Geometry: final body of the model. Coordinates: model frame, mm. Face numbers are marked on the shaded views. A direction names the side the tool comes from. Give positions to 0.01 mm unless a question says otherwise; leave off trailing zeros. Write each loop counter-clockwise with the first axis right and the second up, starting at its lowest first coordinate (ties: lowest second). Pieces come first, ordered by that corner, then holes.
Q1. Cut plane B-B on x = -4. Return the cut outline in (y, z), plus the area to 3 significant figures.
Q2. Cut plane D-D on y = -9.25. Return the cut outline in (x, z), plus the area to 3 significant figures.
Q3. Pin query (flat end, axial travel): pin 1 (10 mm diameter, centred on x = -4, z = -16, fed in from +Y); pin 2 (1 mm diameter, centred on x = -10, z = -24, fed in from -Y); pin 3 (3 mm diameter, centred on y = 8, z = -17, fed in from -X); pin 4 (8 mm diameter, centred on x = -11, y = 3, fed in from +Z). Return the tip coordinate at first contact, or that it passes through.
Q4. Cut plane C-C on y = -2. Return the cut outline in (x, z), plus the area to 3 significant figures.
Q5. Reachability of the marked faces 4, 5 and 6 from +Z, -Z, +X, -X, +Y, -Y: full face, straight path, thin tool, end or side. Return the list, or none.
Q6. Line query: L1, parallel to Y at x = 0, z = -24.5; L2, parallel to Z at x = -4, y = 16.5; L3, parallel to Y at x = -17, z = -4. Output: solid intervals per line, ascending.
Q7. Draft query along Y for the marked faces 1, 2 and 3. Return one class per face: pulls with the +Y half, pulls with the -Y half, needs draft (parallel to the pull), parting line crosses it, or undercut.
Q8. Cut plane A-A on z = -16. Return the cut outline in (x, y).
Autodesk Inventor part; units mm, degrees
ref_plane "Work Plane1" through (-15, 0, -27.5) normal (-1, 0, 0) x (0, -1, 0)
ref_plane "YZ Plane" through (0, 0, 0) normal (1, 0, 0) x (0, 1, 0)
ref_plane "XZ Plane" through (0, 0, 0) normal (0, 1, 0) x (-1, 0, 0)
sketch "Sketch1" plane through (0, 0, 0) normal (0, 1, 0) x (-1, 0, 0)
  line L0 (0, 0) -> (-25, 0)
  line L1 (-25, 0) -> (-25, -10)
  line L2 (-25, -10) -> (-15, -10)
  line L3 (-15, -10) -> (-15, -45)
  line L4 (-15, -45) -> (0, -45)
  line L5 (0, 0) -> (0, -45)
  dimension "d3" = 25
  dimension "d4" = 10
  dimension "d5" = 10
  dimension "d6" = 35
  dimension "d7" = 15
revolve "Revolution1" add sketch "Sketch1" angle 360 about axis through (0, 0, 0) along (0, 0, -1)
sketch "Sketch2" plane through (0, 0, 0) normal (0, 0, 1) x (1, 0, 0)
  line L0 (0, 0) -> (30.242, 0) construction
  line L1 (0, 0.5707) -> (22.435, 0.5707) construction
  circle A0 centre (9.7519, 17.4614) radius 2.25
  circle A1 centre (19.998, 0.2854) radius 2.25
  circle A2 centre (10.2461, -17.1761) radius 2.25
  circle A3 centre (-9.7519, -17.4614) radius 2.25
  circle A4 centre (-19.998, -0.2854) radius 2.25
  circle A5 centre (-10.2461, 17.1761) radius 2.25
  dimension "d12" = 4.5
  dimension "d15" = 360
extrude "Extrusion1" cut sketch "Sketch2" against normal through all
sketch "Sketch3" plane through (0, 0, 0) normal (0, 0, 1) x (1, 0, 0)
  circle A0 centre (0, 0) radius 5.5
  dimension "d19" = 11
extrude "Extrusion2" cut sketch "Sketch3" against normal through all
thread "Thread1"
sketch "Sketch4" plane through (0, 0, 0) normal (0, 0, 1) x (1, 0, 0)
  circle A0 centre (0, 0) radius 25
  line L0 (-17, 0) -> (-17, 18.3303)
  line L1 (-17, 0) -> (-17, -18.3303)
extrude "Extrusion3" cut sketch "Sketch4" against normal blind 15 contours L0 L1 A0 picked at (-18.2676, -10.7318)
ref_plane "Work Plane1" through (-15, 0, -27.5) normal (-1, 0, 0) x (0, -1, 0)
sketch "Sketch5" plane through (-15, 0, -27.5) normal (-1, 0, 0) x (0, -1, 0)
  line L0 (1.9646, 17.5) -> (-2.5354, 17.5)
  line L1 (15, -17.5) -> (-15, -17.5)
  line L2 (0, -11.5) -> (-5, -11.5)
  line L3 (-5.5, 27.5) -> (-5.5, -17.5)
  line L4 (-5, -11.5) -> (-5, 17.5)
  line L5 (15, 17.5) -> (-15, 17.5)
  line L6 (0, -11.5) -> (5, -11.5)
  line L7 (5, -11.5) -> (5, 17.5)
  line L8 (5, 17.5) -> (-5, 17.5)
  point P0 (0, 27.5)
extrude "Extrusion4" cut sketch "Sketch5" against normal blind 1
sketch "Sketch9" plane through (0, 0, -10) normal (0, 0, -1) x (-1, 0, 0)
  line L0 (14, 5) -> (14, -5)
  line L1 (14, 0) -> (22, 0)
  line L2 (22, 0) -> (22, -11.8743)
  line L3 (22, -11.8743) -> (22, 11.8743)
  arc A0 (22, 11.8743) -> (17.2515, 18.0938) centre (0, 0) ccw
  line L4 (17, -18.3303) -> (17, 18.3303)
  line L5 (17, 18.3303) -> (17, -18.3303)
  line L6 (17, 18.3303) -> (17, -18.3303)
  arc A1 (17, -18.3303) -> (22, -11.8743) centre (0, 0) ccw
  arc A2 (22, 11.8743) -> (17, 18.3303) centre (0, 0) ccw
  arc A3 (14.1421, 5) -> (14.1421, -5) centre (0, 0) ccw
  dimension "d59" = 8
extrude "Extrusion5" add sketch "Sketch9" against normal blind 10
sketch "Sketch20" plane through (-14, 0, -27.5) normal (-1, 0, 0) x (0, 0, 1)
  line L0 (17.5, -11.8743) -> (17.5, 11.8743)
  circle A0 centre (11.5, 9.25) radius 3.75
  line L1 (-17.5, -15) -> (-17.5, 15)
  line L2 (11.5, 9.25) -> (-3.7889, -9.25)
  circle A1 centre (-3.7889, -9.25) radius 3.75
  point P0 (27.5, 0)
  dimension "d85" = 7.5
  dimension "d87" = 24
  dimension "d88" = 7.5
extrude "Extrusion8" cut sketch "Sketch20" against normal blind 4.75
sketch "Sketch21" plane through (-22, -11.8743, -10) normal (0, 0, -1) x (-1, 0, 0)
  point P0 (-22, 11.8743)
sketch "Sketch22" plane through (-22, -11.8743, -10) normal (0, 0, -1) x (-1, 0, 0)
  point P0 (-22, 11.8743)
sketch "Sketch23" plane through (-22, -11.8743, -10) normal (0, 0, -1) x (-1, 0, 0)
  arc A0 (-7.8579, 16.8743) -> (-7.8579, 6.8743) centre (-22, 11.8743) ccw
  arc A1 (0, 23.7487) -> (0, 0) centre (-22, 11.8743) ccw
  line L0 (-37, -8.1257) -> (-47.4738, -8.1257)
  line L1 (-47.4738, -8.1257) -> (-47.4738, 31.8346)
  line L2 (-47.4738, 31.8346) -> (-37, 31.8346)
  line L3 (-37, 31.8346) -> (-37, -8.1257)
  line L4 (-22, -13.1257) -> (-22, -11.1257) construction
  line L5 (-31.798, -11.1257) -> (-12.0273, -11.1257)
  line L6 (-12.0273, -11.1257) -> (-12.0273, -17.6927)
  line L7 (-12.0273, -17.6927) -> (-31.798, -17.6927)
  line L8 (-31.798, -17.6927) -> (-31.798, -11.1257)
  line L9 (-22, 11.8743) -> (-7, 11.8743) construction
  line L10 (-31.798, 34.8743) -> (-12.0273, 34.8743)
  line L11 (-12.0273, 34.8743) -> (-12.0273, 41.4414)
  line L12 (-12.0273, 41.4414) -> (-31.798, 41.4414)
  line L13 (-31.798, 41.4414) -> (-31.798, 34.8743)
  dimension "d91" = 2
extrude "Extrusion9" cut sketch "Sketch23" against normal blind 10
properties part number "nut"
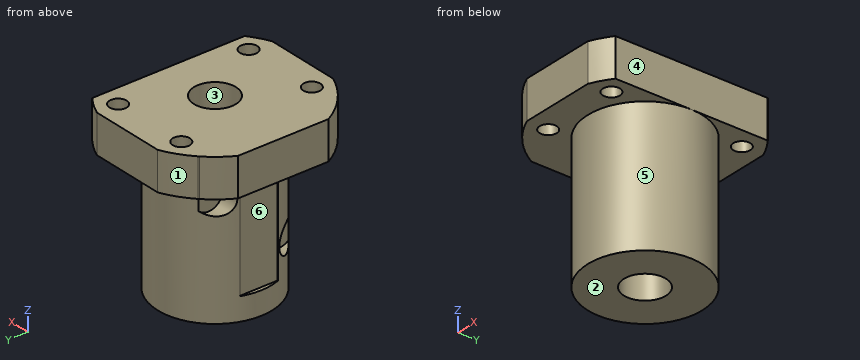
Data:
1. outline: (-23, -10) - (-14.46, -10) - (-14.46, -45) - (-3.77, -45) - (-3.77, 0) - (-23, 0) - close; (3.77, -45) - (14.46, -45) - (14.46, -10) - (23, -10) - (23, 0) - (3.77, 0) - close
1. area: 1,130 mm2
2. outline: (-22, -10) - (-11.81, -10) - (-11.81, -27.54) - (-9.25, -27.54) - (-9.25, -35.04) - (-11.81, -35.04) - (-11.81, -45) - (11.81, -45) - (11.81, -10) - (15, -10) - (15, 0) - (-22, 0) - close
2. area: 1,180 mm2
3. pin 1: stops at y = 15
3. pin 2: stops at y = -11.61
3. pin 3: stops at x = -9.25
3. pin 4: stops at z = 0
4. outline: (-22, -10) - (-14, -10) - (-14, -39) - (-14.87, -39) - (-14.87, -45) - (-5.12, -45) - (-5.12, 0) - (-22, 0) - close; (5.12, -45) - (14.87, -45) - (14.87, -10) - (15, -10) - (15, 0) - (5.12, 0) - close
4. area: 924 mm2
5. face 4: +Z, -Z, +X, -Y
5. face 5: -Z
5. face 6: -X
6. L1: y = -15 to -5.5, 5.5 to 15
6. L2: z = -10 to 0
6. L3: y = -18.33 to 18.33
7. face 1: pulls with the +Y half
7. face 2: needs draft
7. face 3: undercut
8. outline: (-14.14, -5) arc R15 ccw (long way) to (-9.25, 11.81) - (-9.25, 5.5) - (-13.96, 5.5) arc R15 ccw to (-14.14, 5) - (-14, 5) - (-14, -5) - close; hole circle Ø11 at (0, 0)
